from build123d import *

# Parameters (mm, degrees)
EXTRUDE_1_DEPTH = 5


with BuildPart() as part:
    # 草图1 → 凸台-拉伸1 (new body)
    with BuildSketch(Plane(origin=(0, 0, 0), x_dir=(1, 0, 0), z_dir=(0, 1, 0))):
        with BuildLine():
            Line((-21.653867872, 23.131212261), (-41.397029955, -1.695585454))
            ThreePointArc((-41.397029955, -1.695585454), (0, -17.080137941), (41.397029955, -1.695585454))
            Line((41.397029955, -1.695585454), (21.653867872, 23.131212261))
            ThreePointArc((21.653867872, 23.131212261), (0, 14.589673731), (-21.653867872, 23.131212261))
        make_face()
        Polygon((-24.400377301, -6.217451313), (-13.124065852, -10.321693033), (-5.599622699, 10.351544624), (-16.875934148, 14.455786344), align=None, mode=Mode.SUBTRACT)
        Polygon((16.875934148, 14.455786344), (5.599622699, 10.351544624), (13.124065852, -10.321693033), (24.400377301, -6.217451313), align=None, mode=Mode.SUBTRACT)
    extrude(amount=EXTRUDE_1_DEPTH)


solid = part.part
CAD build for the part. Positions are in the model's coordinates, mm. A direction names the side the tool comes from. Give positions to 0.01 mm unless a question says otherwise; leave off trailing zeros. Write each loop counter-clockwise with the first axis right and the second up, starting at its lowest first coordinate (ties: lowest second). Pieces come first, ordered by that corner, then holes. Notation, with made-up numbers: (84, 27) -> (96, 27) arc R25 cw to (96, 65) -> close; hole circle Ø9 at (0, 67). An arc over 180 degrees is marked (long way). Return JSON: item names as keys, results as strings.
Item 1: Band-saw the part on B-B (y = 1.4). List the corners of the cut face in (x, z).
Answer below:
{"outline": "(-41.4, 1.7) -> (-21.65, -23.13) arc R31.72 cw to (21.65, -23.13) -> (41.4, 1.7) arc R63.39 ccw to start; hole (-24.4, 6.22) -> (-16.88, -14.46) -> (-5.6, -10.35) -> (-13.12, 10.32) -> close; hole (5.6, -10.35) -> (16.88, -14.46) -> (24.4, 6.22) -> (13.12, 10.32) -> close"}
Item 2: Band-saw the part on D-D (z = -18). List the corners of the cut face in (x, y), then the cut area to 3 significant figures.
Answer below:
{"outline": "(-25.73, 0) -> (-14.31, 0) -> (-14.31, 5) -> (-25.73, 5) -> close; (14.31, 0) -> (25.73, 0) -> (25.73, 5) -> (14.31, 5) -> close", "area": "114 mm2"}
Item 3: Tool access for faces 4 (the flat face through (-18.84, 2.46, 8.24)), 5 (the cylindrical face through (-0.632, 2.465, 17.077)): list every direction of +Z, -Z, +X, -X, +Y, -Y with a clear straight run to the whole face (end or side of a thin tool).
Answer below:
{"face 4": "+Y, -Y", "face 5": "+Z, +Y, -Y"}
Item 4: Drill centre lines: probe 1 along X at (y, z) = (2.6, -1.5); probe 2 along X at (y, z) = (4.4, -2); probe 3 along X at (y, z) = (1.15, -20). Where is each one in solid material? Low to high.
Answer below:
{"probe 1": "x = -38.86 to -21.59, -8.82 to 8.82, 21.59 to 38.86", "probe 2": "x = -38.46 to -21.41, -8.64 to 8.64, 21.41 to 38.46", "probe 3": "x = -24.14 to -17.72, 17.72 to 24.14"}
Item 5: Band-saw the part on C-C (x = 16). List the corners of the cut face in (y, z), then the cut area to 3 significant figures.
Answer below:
{"outline": "(0, -18.92) -> (5, -18.92) -> (5, -14.14) -> (0, -14.14) -> close; (0, 9.27) -> (5, 9.27) -> (5, 15.03) -> (0, 15.03) -> close", "area": "52.7 mm2"}
Item 6: Two-plate mould, pull along Z, no slides. Class faces 1 (the flat face through (-31.39, 2.46, -10.89)), 2 (the flat face through (-1, 0, 1)), 3 (the flat face through (-11.159, 2.465, -12.375)): +Z half, -Z half, draft (parallel to the pull), parting line (faces both ways), or undercut.
Answer below:
{"face 1": "-Z half", "face 2": "draft", "face 3": "undercut"}
Item 7: Band-saw the part on A-A (z = -7). List the corners of the cut face in (x, y).
Answer below:
{"outline": "(-34.48, 0) -> (-19.59, 0) -> (-19.59, 5) -> (-34.48, 5) -> close; (-6.82, 0) -> (6.82, 0) -> (6.82, 5) -> (-6.82, 5) -> close; (19.59, 0) -> (34.48, 0) -> (34.48, 5) -> (19.59, 5) -> close"}
